Source: three-view drawing plus pictorial views. Frame: mm from the lowest corner of the part. A direction names the side the tool comes from. Give positions to 0.01 mm unless a question says otherwise; leave off trailing zeros. Order: outer loops, then holes, each group sorted by start corner. A loop starts at its lowest first (then second) coordinate and runs counter-clockwise, first axis right, second up. Notation, with made-up numbers: (29.5, 26) -> (37.5, 26) arc R19 cw to (37.5, 52) -> close; hole circle Ø10 at (15.25, 46.25). An arc over 180 degrees is marked (long way). Write item = value, one per line.
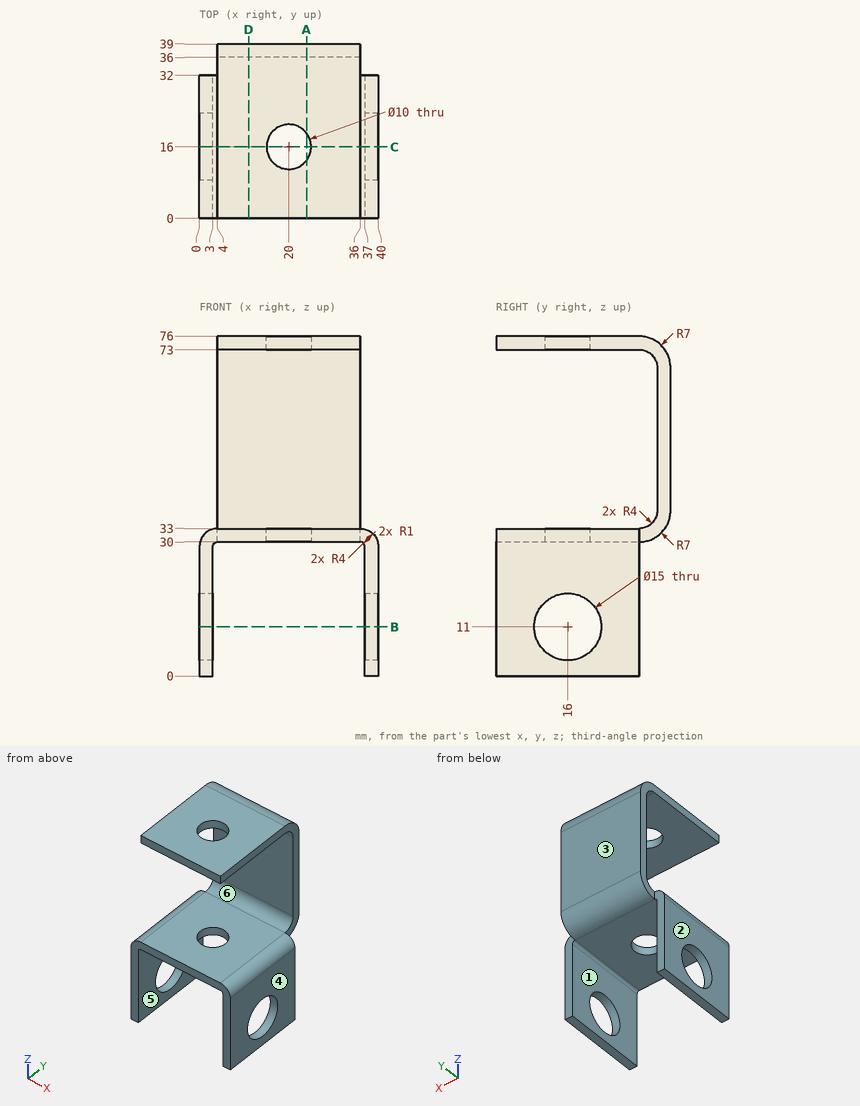
1) Section query C-C (y = 16). Count the separate pieces of the cut face and the enclosed holes in it, plus the area to 3 significant figures.
Check sheet entries:
separate_pieces = 6
enclosed_holes = 0
area = 240 mm²
2) Mould query, pull axis X, two halves, no side actions, for the marked faces 1, 2 and 3. Classes: +X half, -X half, draft (parallel to the pull), parting line (faces both ways), or undercut.
Check sheet entries:
face_1 = undercut
face_2 = -X half
face_3 = draft
3) Line query: line 1 (X direction, y = 27.5, z = 29); line 2 (Z direction, x = 34.5, y = 31); line 3 (Y direction, x = 1, z = 11). Output: solid intervals per line, ascending. Write a range as from..to.
Check sheet entries:
line_1 = 0..3, 37..40
line_2 = 30..33, 73..76
line_3 = 0..8.5, 23.5..32
4) Section query B-B (z = 11). Output: boundary loops of the cut face in (x, y).
Check sheet entries:
outline = (0, 0) -> (3, 0) -> (3, 8.5) -> (0, 8.5) -> close; (0, 23.5) -> (3, 23.5) -> (3, 32) -> (0, 32) -> close; (37, 0) -> (40, 0) -> (40, 8.5) -> (37, 8.5) -> close; (37, 23.5) -> (40, 23.5) -> (40, 32) -> (37, 32) -> close
5) Section query D-D (x = 11). Output: boundary loops of the cut face in (y, z).
Check sheet entries:
outline = (0, 30) -> (32, 30) arc R7 ccw to (39, 37) -> (39, 69) arc R7 ccw to (32, 76) -> (0, 76) -> (0, 73) -> (32, 73) arc R4 cw to (36, 69) -> (36, 37) arc R4 cw to (32, 33) -> (0, 33) -> close
6) Reachability of the marked faces 4, 5 and 6 from +Z, -Z, +X, -X, +Y, -Y: full face, straight path, thin tool, end or side. Return the list, or none.
Check sheet entries:
face_4 = +Z, -Z, +X, +Y, -Y
face_5 = -Z, +Y, -Y
face_6 = +X, -X, -Y
7) First-contact query: P1, Ø10, axis at y = 29, z = 36, coming from the +X side; P2, Ø2, axis at x = 39, z = 10.5, coming from the +Y side; P3, Ø9.5, axis at x = 26, y = 23, coming from the -Z side; P4, Ø8, axis at x = 19, y = 33.5, coming from the +Z side. Flat tips, straight axial feed; report the tip coordinate or a pass-through.
Check sheet entries:
P1 = 39.46
P2 = 32
P3 = 30
P4 = 76
8) Section query A-A (x = 24). Output: boundary loops of the cut face in (y, z), plus the area to 3 significant figures.
Check sheet entries:
outline = (0, 30) -> (13, 30) -> (13, 33) -> (0, 33) -> close; (0, 73) -> (13, 73) -> (13, 76) -> (0, 76) -> close; (19, 30) -> (32, 30) arc R7 ccw to (39, 37) -> (39, 69) arc R7 ccw to (32, 76) -> (19, 76) -> (19, 73) -> (32, 73) arc R4 cw to (36, 69) -> (36, 37) arc R4 cw to (32, 33) -> (19, 33) -> close
area = 304 mm²
